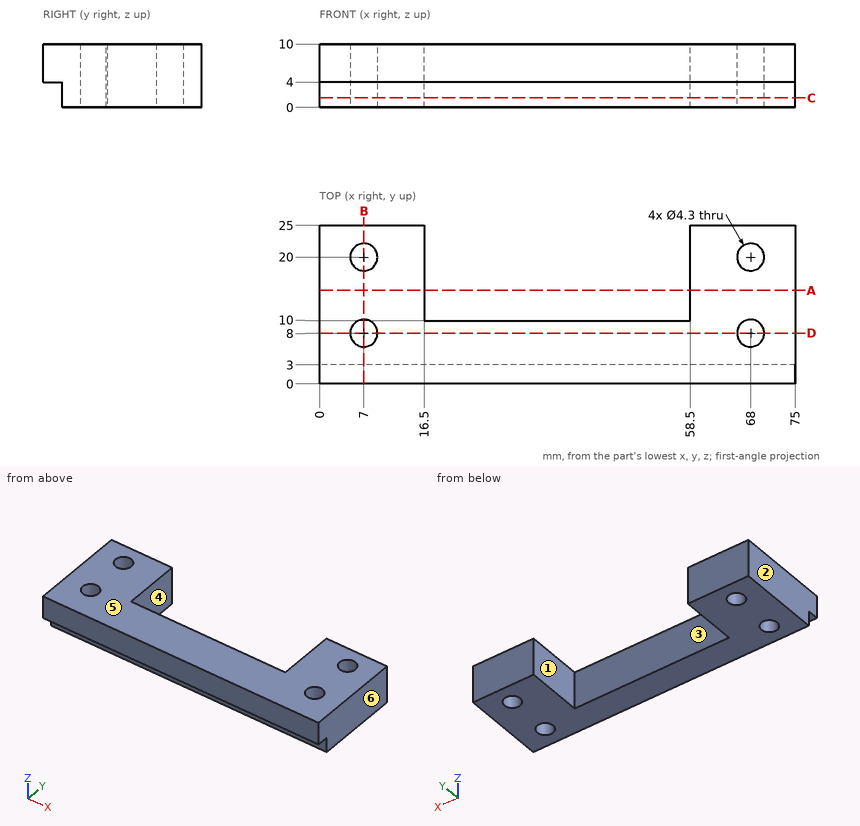
Geometry check sheet. Reference: drawing and pictorial views, mm from the part's lowest x, y, z. A direction names the side the tool comes from. Give positions to 0.01 mm unless a question says otherwise; leave off trailing zeros. Write each loop counter-clockwise with the first axis right and the second up, starting at its lowest first coordinate (ties: lowest second). Pieces come first, ordered by that corner, then holes. Notation, with made-up numbers: (-30.5, 28.25) -> (-10.5, 28.25) arc R21 cw to (-10.5, 41.25) -> close; hole circle Ø5 at (63.5, -32). An arc over 180 degrees is marked (long way). One line per question, with ' | ' between items.
Item 1: Access from +Z, -Z, +X, -X, +Y, -Y to the whole of each face (thin tool, end or side, straight path). Record for the marked faces 1 and 2.
Determined:
face 1: +Z, -Z, +Y | face 2: +Z, -Z, -X, +Y, -Y
Item 2: Sectioned sample at A-A, the plane y = 14.75. Record the boundary of the cut face in (x, z).
Determined:
outline: (0, 0) -> (16.5, 0) -> (16.5, 10) -> (0, 10) -> close; (58.5, 0) -> (75, 0) -> (75, 10) -> (58.5, 10) -> close
Item 3: Sectioned sample at C-C, the plane z = 1.5. Record the boundary of the cut face in (x, y).
Determined:
outline: (0, 3) -> (75, 3) -> (75, 25) -> (58.5, 25) -> (58.5, 10) -> (16.5, 10) -> (16.5, 25) -> (0, 25) -> close; hole circle Ø4.3 at (7, 8); hole circle Ø4.3 at (7, 20); hole circle Ø4.3 at (68, 8); hole circle Ø4.3 at (68, 20)
Item 4: Draft check along X on the marked faces 3, 4, 5 and 6. Enter one of: released by +X, released by -X, zero draft, split by the parting line, or undercut.
Determined:
face 3: undercut | face 4: undercut | face 5: zero draft | face 6: released by +X
Item 5: Sectioned sample at D-D, the plane y = 8. Record the boundary of the cut face in (x, z), plus the area to 3 significant figures.
Determined:
outline: (0, 0) -> (4.85, 0) -> (4.85, 10) -> (0, 10) -> close; (9.15, 0) -> (65.85, 0) -> (65.85, 10) -> (9.15, 10) -> close; (70.15, 0) -> (75, 0) -> (75, 10) -> (70.15, 10) -> close | area: 664 mm^2
Item 6: Depth check by flat-ended pin: pin 1 (6 mm diameter, centred on x = 52, y = 5, fed in from -Z); pin 2 (2.5 mm diameter, centred on x = 48, y = 1, fed in from -Z); pin 3 (5 mm diameter, centred on x = 30.5, z = 4, fed in from +Y); pin 4 (2.5 mm diameter, centred on x = 7, y = 8, fed in from -Z). Enter the tip coordinate at first touch or a pass-through.
Determined:
pin 1: z = 0 | pin 2: z = 4 | pin 3: y = 10 | pin 4: through
Item 7: Sectioned sample at B-B, the plane x = 7. Record the boundary of the cut face in (y, z), plus the area to 3 significant figures.
Determined:
outline: (0, 4) -> (3, 4) -> (3, 0) -> (5.85, 0) -> (5.85, 10) -> (0, 10) -> close; (10.15, 0) -> (17.85, 0) -> (17.85, 10) -> (10.15, 10) -> close; (22.15, 0) -> (25, 0) -> (25, 10) -> (22.15, 10) -> close | area: 152 mm^2
Item 8: Scan lines: line 1 along Y through (x, z) = (68, 7.25); line 2 along Y through (x, z) = (68, 3.5); line 3 along X through (y, z) = (19.75, 5.25). Record each from-to range of solid material in increasing order.
Determined:
line 1: 0 to 5.85, 10.15 to 17.85, 22.15 to 25 | line 2: 3 to 5.85, 10.15 to 17.85, 22.15 to 25 | line 3: 0 to 4.86, 9.14 to 16.5, 58.5 to 65.86, 70.14 to 75
